Verification items for the finished model (mm, model axes). A direction names the side the tool comes from. Give positions to 0.01 mm unless a question says otherwise; leave off trailing zeros. Loops run counter-clockwise (first coordinate to the right, second up) from the corner with the lowest first, then second, coordinate; pieces in that order, holes last. Notation, with made-up numbers: (28, 41) - (53, 41) arc R18 cw to (53, 72) - close; hole circle Ø2 at (45.5, 5). An arc over 180 degrees is marked (long way). One line per item, written item: value. Start each with the question number.
1. Access from +Z, -Z, +X, -X, +Y, -Y to the whole of each face (thin tool, end or side, straight path). Record for faces 1 (the cylindrical face through (0, 2, -2)), 2 (the flat face through (0, 0, 15)), 3 (the flat face through (0, -4.33, 15)).
2. Sectioned sample at B-B (y = -0.75). Record the cut outline in (x, z), plus the area to 3 significant figures.
3. Scan lines: L1, parallel to Y at x = 0, z = 21; L2, parallel to Z at x = 2.75, y = 1.25; L3, parallel to Z at x = 1.25, y = 0.25. Record each from-to range of solid material in increasing order. Write a range as [from, to].
4. Sectioned sample at C-C (y = -3). Record the cut outline in (x, z), plus the area to 3 significant figures.
5. Sectioned sample at D-D (x = 4). Record the cut outline in (y, z).
6. Gauge pin test, flat ends, axial feed: pin 1 (1.2 mm diameter, centred on x = -0.5, y = 0, fed in from +Z); pin 2 (2 mm diameter, centred on y = -3, z = 7.5, fed in from -X); pin 3 (3 mm diameter, centred on y = 1, z = 23.5, fed in from +X). Record the tip position at first contact, or that the pin passes through.
7. Sectioned sample at A-A (x = 0). Record the cut outline in (y, z).
8. Mould release check, pull along Y, two halves, no side actions. Record for faces 4 (the flat face through (2.2, 0.1, 0)), 5 (the flat face through (3.77, 2.13, 14.79)), 6 (the flat face through (-3.77, -2.13, 14.79)), 7 (the cylindrical face through (0, -2, 23)): pulls with the +Y half, pulls with the -Y half, needs draft (parallel to the pull), parting line crosses it, or undercut.
from build123d import *

# Parameters (mm, degrees)
EXTRUDE002_DEPTH = 30
SKETCH010_R      = 2
POCKET002_DEPTH  = 15
SKETCH011_R      = 2
EXTRUDE004_DEPTH = 5


with BuildPart() as pocket002:
    # Sketch008 → Extrude002 (new body)
    with BuildSketch(Plane.XY):
        Polygon((5, 0), (2.5, 4.330127), (-2.5, 4.330127), (-5, 0), (-2.5, -4.330127), (2.5, -4.330127), align=None)
    extrude(amount=EXTRUDE002_DEPTH)

    # Sketch010 → Pocket002 (cut)
    with BuildSketch(Plane.XY.offset(30)):
        Circle(SKETCH010_R)
    extrude(amount=-POCKET002_DEPTH, mode=Mode.SUBTRACT)


with BuildPart() as obj1:
    # Sketch011 → Extrude004 (new body)
    with BuildSketch(Plane(origin=(0, 0, 0), x_dir=(1, 0, 0), z_dir=(0, 0, -1))):
        Circle(SKETCH011_R)
    extrude(amount=EXTRUDE004_DEPTH)

    # Fusion: union Pocket002
    add(pocket002.part)


solid = obj1.part
Results are:
1. face 1: -Z
1. face 2: +Z
1. face 3: +Z, -Z, +X, -X, -Y
2. outline: (-4.57, 0) - (-1.85, 0) - (-1.85, -5) - (1.85, -5) - (1.85, 0) - (4.57, 0) - (4.57, 30) - (1.85, 30) - (1.85, 15) - (-1.85, 15) - (-1.85, 30) - (-4.57, 30) - close
2. area: 237 mm^2
3. L1: y = [-4.33, -2], [2, 4.33]
3. L2: z = [0, 30]
3. L3: z = [-5, 15]
4. outline: (-3.27, 0) - (3.27, 0) - (3.27, 30) - (-3.27, 30) - close
4. area: 196 mm^2
5. outline: (-1.73, 0) - (1.73, 0) - (1.73, 30) - (-1.73, 30) - close
6. pin 1: stops at z = 15
6. pin 2: stops at x = -3.85
6. pin 3: stops at x = 5
7. outline: (-4.33, 0) - (-2, 0) - (-2, -5) - (2, -5) - (2, 0) - (4.33, 0) - (4.33, 30) - (2, 30) - (2, 15) - (-2, 15) - (-2, 30) - (-4.33, 30) - close
8. face 4: needs draft
8. face 5: pulls with the +Y half
8. face 6: pulls with the -Y half
8. face 7: undercut
